Read the model definition and answer for the solid it produces. Units are mm, in the model's axes. A direction names the side the tool comes from. Round coordinates to 2 decimals unless told otherwise and drop trailing zeros. Order: outer loops, then holes, each group sorted by start corner. A loop starts at its lowest first (then second) coordinate and runs counter-clockwise, first axis right, second up.
from build123d import *

# Parameters (mm, degrees)
SKETCH_1_W      = 5
SKETCH_1_H      = 40
EXTRUDE_1_DEPTH = 1


with BuildPart() as part:
    # 草图1 → 凸台-拉伸1 (new, symmetric)
    with BuildSketch(Plane.XY):
        with BuildLine():
            Line((2, 0), (2, -9))
            ThreePointArc((2, -9), (5, -12), (8, -9))
            Line((8, -9), (8, 0))
            Line((8, 0), (62, 0))
            Line((62, 0), (62, -9))
            ThreePointArc((62, -9), (65, -12), (68, -9))
            Line((68, -9), (68, 0))
            Line((68, 0), (70, 0))
            Line((70, 0), (70, 60))
            Line((70, 60), (68, 60))
            Line((68, 60), (68, 69))
            ThreePointArc((68, 69), (65, 72), (62, 69))
            Line((62, 69), (62, 60))
            Line((62, 60), (8, 60))
            Line((8, 60), (8, 69))
            ThreePointArc((8, 69), (5, 72), (2, 69))
            Line((2, 69), (2, 60))
            Line((2, 60), (0, 60))
            Line((0, 60), (0, 0))
            Line((0, 0), (2, 0))
        make_face()
        with Locations((12.5, 30)):
            Rectangle(SKETCH_1_W, SKETCH_1_H, mode=Mode.SUBTRACT)
        with Locations((27.5, 30)):
            Rectangle(SKETCH_1_W, SKETCH_1_H, mode=Mode.SUBTRACT)
        with Locations((42.5, 30)):
            Rectangle(SKETCH_1_W, SKETCH_1_H, mode=Mode.SUBTRACT)
        with Locations((57.5, 30)):
            Rectangle(SKETCH_1_W, SKETCH_1_H, mode=Mode.SUBTRACT)
    extrude(amount=EXTRUDE_1_DEPTH, both=True)


solid = part.part
Q1. A cutting plane is placed at C-C, the plane z = 0.1. Give the number of separate pieces and of enclosed holes in the cut face, plus the area to 3 significant figures.
Outcome:
separate pieces: 1
enclosed holes: 4
area: 3,670 mm2
Q2. Flat-ended cylindrical pins translate along their axes: pin 1 (0.6 mm diameter, centred on y = 62.5, z = -0.5, fed in from -X); pin 2 (0.6 mm diameter, centred on y = 25, z = 0.5, fed in from -X); pin 3 (1 mm diameter, centred on x = 28.5, z = 0.5, fed in from +Y). Find the tip coordinate at first contact, or state that the pin passes through.
Outcome:
pin 1: stops at x = 2
pin 2: stops at x = 0
pin 3: stops at y = 60
Q3. Straight lines are drawn through the part: probe 1 along X at (y, z) = (10.5, 0.5); probe 2 along Y at (x, z) = (13.5, 0.55); probe 3 along X at (y, z) = (67.5, 0.9). For each, find the intervals that lie inside material, in ascending order.
Outcome:
probe 1: x = 0 to 10, 15 to 25, 30 to 40, 45 to 55, 60 to 70
probe 2: y = 0 to 10, 50 to 60
probe 3: x = 2 to 8, 62 to 68
Q4. A cutting plane is placed at B-B, the plane x = 28. Give the vertices of the cut face in (y, z), plus the area to 3 significant figures.
Outcome:
outline: (0, -1) - (10, -1) - (10, 1) - (0, 1) - close; (50, -1) - (60, -1) - (60, 1) - (50, 1) - close
area: 40.0 mm2
Q5. For faces 1 (the face through (69, 60, 0)), 2 (the face through (55, 30, 0)), 3 (the face through (1, 0, 0)), determine the directions among +Z, -Z, +X, -X, +Y, -Y from which every point of the face is accessible in a straight line to the end or side of a thin tool.
Outcome:
face 1: +Z, -Z, +X, +Y
face 2: +Z, -Z
face 3: +Z, -Z, -X, -Y
Q6. For a pull along X with two mould halves and no side action, classify faces 4 (the face through (57, 50, 0)), 5 (the face through (1, 60, 0)), 6 (the face through (68, 64, 0)) as released by +X, released by -X, zero draft, split by the parting line, or undercut.
Outcome:
face 4: undercut
face 5: zero draft
face 6: released by +X
Q7. A cutting plane is placed at A-A, the plane y = 13. Give the vertices of the cut face in (x, z).
Outcome:
outline: (0, -1) - (10, -1) - (10, 1) - (0, 1) - close; (15, -1) - (25, -1) - (25, 1) - (15, 1) - close; (30, -1) - (40, -1) - (40, 1) - (30, 1) - close; (45, -1) - (55, -1) - (55, 1) - (45, 1) - close; (60, -1) - (70, -1) - (70, 1) - (60, 1) - close
